Check sheet for the modelled part. Datum: model origin and axes. Units: mm. A direction names the side the tool comes from. Give positions to 0.01 mm unless a question says otherwise; leave off trailing zeros. Write each loop counter-clockwise with the first axis right and the second up, starting at its lowest first coordinate (ties: lowest second). Pieces come first, ordered by that corner, then holes. Notation, with made-up numbers: (22.5, 24.5) -> (38.5, 24.5) arc R27 ccw to (38.5, 49.5) -> close; hole circle Ø4 at (-23, 45.5). An arc over 180 degrees is marked (long way). Return JSON: item names as keys, results as strings.
from build123d import *

# Parameters (mm, degrees)
F0_W     = 120
F0_H     = 60
F1_DEPTH = 150
F2_W     = 142
F2_H     = 116
F3_DEPTH = 56
F4_W     = 5
F4_H     = 60
F5_DEPTH = 2
F6_W     = 5
F6_H     = 60
F7_DEPTH = 2
F8_W     = 146
F8_H     = 5
F9_DEPTH = 2


with BuildPart() as f1:
    # F0 (on Right) → F1 (new body)
    with BuildSketch(Plane.YZ):
        with Locations((-60, 30)):
            Rectangle(F0_W, F0_H)
    extrude(amount=-F1_DEPTH)

    # F2 (on face) → F3 (cut)
    with BuildSketch(Plane.XY.offset(60)):
        with Locations((-75, -62)):
            Rectangle(F2_W, F2_H)
    extrude(amount=-F3_DEPTH, mode=Mode.SUBTRACT)

    # F4 (on face) → F5 (cut)
    with BuildSketch(Plane(origin=(-150, 0, 0), x_dir=(0, -1, 0), z_dir=(-1, 0, 0))):
        with Locations((117.5, 30)):
            Rectangle(F4_W, F4_H)
    extrude(amount=-F5_DEPTH, mode=Mode.SUBTRACT)

    # F6 (on face) → F7 (cut)
    with BuildSketch(Plane.YZ):
        with Locations((-117.5, 30)):
            Rectangle(F6_W, F6_H)
    extrude(amount=-F7_DEPTH, mode=Mode.SUBTRACT)

    # F8 (on face) → F9 (cut)
    with BuildSketch(Plane(origin=(0, 0, 0), x_dir=(1, 0, 0), z_dir=(0, 0, -1))):
        with Locations((-75, 117.5)):
            Rectangle(F8_W, F8_H)
    extrude(amount=-F9_DEPTH, mode=Mode.SUBTRACT)


solid = f1.part
(1) Depth check by flat-ended pin: pin 1 Ø1.5 at (y, z) = (-118, 45) entering from +X; pin 2 Ø12 at (x, z) = (-58, 33) entering from -Y; pin 3 Ø4 at (x, y) = (-81, -24) entering from +Z. Enter the tip coordinate at first touch or a pass-through.
Reply:
{"pin 1": "x = -2", "pin 2": "y = -4", "pin 3": "z = 4"}
(2) Cross-section at A-A on x = -105. Enter the section's corners in (y, z), then the cut area to 3 significant figures.
Reply:
{"outline": "(-120, 2) -> (-115, 2) -> (-115, 0) -> (0, 0) -> (0, 60) -> (-4, 60) -> (-4, 4) -> (-120, 4) -> close", "area": "694 mm^2"}
(3) Cross-section at C-C on z = 21.5. Enter the section's corners in (x, y), then the cut area to 3 significant figures.
Reply:
{"outline": "(-150, -115) -> (-148, -115) -> (-148, -120) -> (-146, -120) -> (-146, -4) -> (-4, -4) -> (-4, -120) -> (-2, -120) -> (-2, -115) -> (0, -115) -> (0, 0) -> (-150, 0) -> close", "area": "1,510 mm^2"}
(4) Release check for a two-part mould opening along X. For faces 1 (the flat face through (-75, -115, 1)), 2 (the flat face through (-76, -61, 4)), 3 (the flat face through (-150, -58, 30)) record: pulls with the +X half, pulls with the -X half, needs draft (parallel to the pull), parting line crosses it, or undercut.
Reply:
{"face 1": "needs draft", "face 2": "undercut", "face 3": "pulls with the -X half"}
(5) Cross-section at B-B on y = -9.5. Enter the section's corners in (x, z).
Reply:
{"outline": "(-150, 0) -> (0, 0) -> (0, 60) -> (-4, 60) -> (-4, 4) -> (-146, 4) -> (-146, 60) -> (-150, 60) -> close"}
(6) Set-up check for faces 4 (the flat face through (-76, -118, 2)), 5 (the flat face through (-4, -63, 32)), 6 (the flat face through (-148, -117, 31)): record each of +Z, -Z, +X, -X, +Y, -Y from which the full face is reachable in a straight line by a thin tool's end or side.
Reply:
{"face 4": "-Z, +X, -X, -Y", "face 5": "+Z, -Y", "face 6": "+Z, -Z, -X, -Y"}
(7) Thickness scan on L1, parallel to X at y = -80, z = 27; L2, parallel to Y at x = -73.5, z = 33.5; L3, parallel to Z at x = -86, y = -108. Record the ranges inside material, lowest first.
Reply:
{"L1": "-150 to -146, -4 to 0", "L2": "-4 to 0", "L3": "0 to 4"}
